Here's how the part is built. I have some questions about the finished solid (model axes, mm). A direction names the side the tool comes from. Coordinates: 2 decimals unless noted, no trailing zeros. Write each loop counter-clockwise with the first axis right and the second up, starting at its lowest first coordinate (ties: lowest second). Pieces come first, ordered by that corner, then holes. Notation, with made-up numbers: (-35, -37) - (11, -37) arc R27 ccw to (11, -13) - close; hole circle Ø5 at (60, 15). An arc over 180 degrees is marked (long way). Answer in a Markdown table with one row per item. Add a question column.
Item 1: Imagine slicing it at C-C (z = -10.5). State how many separate pieces and enclosed holes the cut face has, plus the area to 3 significant figures.
Item 2: Imagine slicing it at A-A (y = 8.5). Please give me the cut outline in (x, z) (3 decimals), plus the area to 3 significant figures.
Item 3: Imagine slicing it at D-D (x = 45). Please give me the cut outline in (y, z).
Item 4: Imagine slicing it at B-B (x = -27). Please give me the cut outline in (y, z) (3 decimals), plus the area to 3 significant figures.
Item 5: I'm going to push flat-ended pins straight in: pin 1 (6 mm diameter, centred on x = 18, z = 1.5, fed in from +Y); pin 2 (13 mm diameter, centred on x = -51, z = -1.5, fed in from +Y). Where does each tip first touch, or does it pass through?
Item 6: Which directions (+Z, -Z, +X, -X, +Y, -Y) give clear straight access to the entire face, cutting with the end or side of a thin tool? Please do faces 1 (the face through (-39.063, 0.493, -0.531)), 2 (the face through (-42, 1, 4)).
Item 7: If I drill on probe 1 along X at (y, z) = (7.75, 0) (3 decimals); probe 2 along X at (y, z) = (7.75, 5); probe 3 along Z at (x, y) = (27, 0.35) (3 decimals), over which ranges is the centre line in solid material (lowest first)? Write a range as from..to.
Item 8: We'd pull the mould along Z, two halves only. Please class faces 3 (the face through (-1, 5, 15)), 4 (the face through (-10, 10, 9)), 5 (the face through (-66.063, 0.493, -0.531)): +Z half, -Z half, draft (parallel to the pull), parting line (faces both ways), or undercut.
from build123d import *

# Parameters (mm, degrees)
ESQUISSE1_W                    = 27
ESQUISSE1_H                    = 30
ESQUISSE1_R                    = 13.075
BOSS_EXTRU_1_DEPTH             = 10
ESQUISSE4_R                    = 13.075
ESQUISSE4_R_2                  = 12.075
BOSS_EXTRU_2_DEPTH             = 1
R_P_TITION_LIN_AIRE1_COUNT     = 3
R_P_TITION_LIN_AIRE1_PITCH     = 27
R_P_TITION_LIN_AIRE1_COL_COUNT = 3
R_P_TITION_LIN_AIRE1_COL_PITCH = 27


with BuildPart() as part:
    # Esquisse1 → Boss.-Extru.1 (new body)
    with BuildSketch(Plane(origin=(0, 0, 0), x_dir=(1, 0, 0), z_dir=(0, 1, 0))):
        Rectangle(ESQUISSE1_W, ESQUISSE1_H)
        Circle(ESQUISSE1_R, mode=Mode.SUBTRACT)
    boss_extru_1 = extrude(amount=BOSS_EXTRU_1_DEPTH)

    # Esquisse4 → Boss.-Extru.2 (add)
    with BuildSketch(Plane(origin=(0, 0, 0), x_dir=(1, 0, 0), z_dir=(0, 1, 0))):
        Circle(ESQUISSE4_R)
        Circle(ESQUISSE4_R_2, mode=Mode.SUBTRACT)
    boss_extru_2 = extrude(amount=BOSS_EXTRU_2_DEPTH)

    # Répétition linéaire1: Boss.-Extru.1, Boss.-Extru.2 ×3
    with Locations(*[(i * R_P_TITION_LIN_AIRE1_PITCH, 0, 0) for i in range(1, R_P_TITION_LIN_AIRE1_COUNT)]):
        add(boss_extru_1)
        add(boss_extru_2)

    # Répétition linéaire1 col: Boss.-Extru.1, Boss.-Extru.2 ×3
    with Locations(*[(-i * R_P_TITION_LIN_AIRE1_COL_PITCH, 0, 0) for i in range(1, R_P_TITION_LIN_AIRE1_COL_COUNT)]):
        add(boss_extru_1)
        add(boss_extru_2)


solid = part.part
Here are the results:
| question | item | result |
|---|---|---|
| 1 | separate pieces | 6 |
| 1 | enclosed holes | 0 |
| 1 | area | 589 mm2 |
| 2 | outline | (-67.5, -15) - (67.5, -15) - (67.5, 15) - (-67.5, 15) - close; hole circle Ø26.15 at (-54, 0); hole circle Ø26.15 at (-27, 0); hole circle Ø26.15 at (0, 0); hole circle Ø26.15 at (27, 0); hole circle Ø26.15 at (54, 0) |
| 2 | area | 1,360 mm2 |
| 3 | outline | (0, -15) - (10, -15) - (10, -9.48) - (1, -9.48) - (1, -8.05) - (0, -8.05) - close; (0, 8.05) - (1, 8.05) - (1, 9.48) - (10, 9.48) - (10, 15) - (0, 15) - close |
| 4 | outline | (0, -15) - (10, -15) - (10, -13.075) - (1, -13.075) - (1, -12.075) - (0, -12.075) - close; (0, 12.075) - (1, 12.075) - (1, 13.075) - (10, 13.075) - (10, 15) - (0, 15) - close |
| 4 | area | 40.5 mm2 |
| 5 | pin 1 | stops at y = 1 |
| 5 | pin 2 | passes through |
| 6 | face 1 | +Y, -Y |
| 6 | face 2 | +Y |
| 7 | probe 1 | x = -67.5..-67.075, -40.925..-40.075, -13.925..-13.075, 13.075..13.925, 40.075..40.925, 67.075..67.5 |
| 7 | probe 2 | x = -67.5..-66.08, -41.92..-39.08, -14.92..-12.08, 12.08..14.92, 39.08..41.92, 66.08..67.5 |
| 7 | probe 3 | z = -15..-12.075, 12.075..15 |
| 8 | face 3 | +Z half |
| 8 | face 4 | draft |
| 8 | face 5 | undercut |
